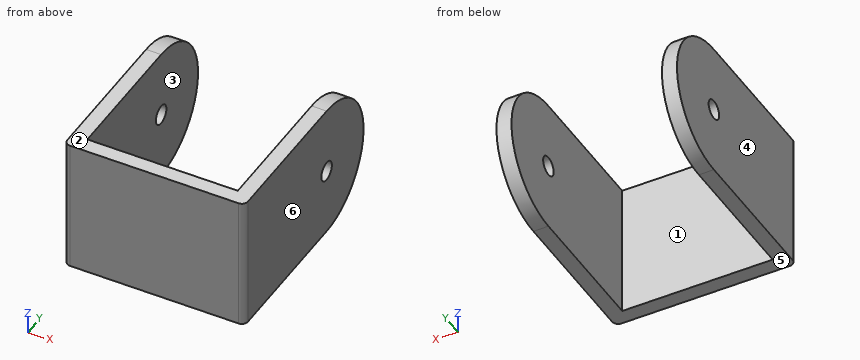
from build123d import *

# Parameters (mm, degrees)
BOSS_EXTRUDE1_DEPTH = 2.5
SKETCH2_W           = 27.5
SKETCH2_H           = 22.5
BOSS_EXTRUDE2_DEPTH = 2.5
SKETCH5_W           = 22.5
SKETCH5_H           = 25
BOSS_EXTRUDE3_DEPTH = 2.5
SKETCH6_R           = 1.6
CUT_EXTRUDE1_DEPTH  = 30
FILLET1_R           = 1


with BuildPart() as part:
    # Sketch1 → Boss-Extrude1 (new body)
    with BuildSketch(Plane(origin=(0, 0, 0), x_dir=(0, 0, -1), z_dir=(1, 0, 0))):
        with BuildLine():
            Line((-11.25, 0), (-11.25, -22.5))
            Line((-11.25, -22.5), (11.25, -22.5))
            Line((11.25, -22.5), (11.25, 0))
            ThreePointArc((11.25, 0), (0, 11.25), (-11.25, 0))
        make_face()
    extrude(amount=BOSS_EXTRUDE1_DEPTH)

    # Sketch2 → Boss-Extrude2 (add)
    with BuildSketch(Plane(origin=(0, -22.5, 0), x_dir=(-1, 0, 0), z_dir=(0, -1, 0))):
        with Locations((-13.75, 0)):
            Rectangle(SKETCH2_W, SKETCH2_H)
    extrude(amount=BOSS_EXTRUDE2_DEPTH)

    # Sketch5 → Boss-Extrude3 (add)
    with BuildSketch(Plane(origin=(27.5, 0, 0), x_dir=(0, 0, -1), z_dir=(1, 0, 0))):
        with BuildLine():
            ThreePointArc((-11.25, 0), (0, 11.25), (11.25, 0))
            Line((11.25, 0), (-11.25, 0))
        make_face()
        with Locations((0, -12.5)):
            Rectangle(SKETCH5_W, SKETCH5_H)
    extrude(amount=BOSS_EXTRUDE3_DEPTH)

    # Sketch6 → Cut-Extrude1 (cut)
    with BuildSketch(Plane(origin=(30, 0, 0), x_dir=(0, 0, -1), z_dir=(1, 0, 0))):
        Circle(SKETCH6_R)
    extrude(amount=-CUT_EXTRUDE1_DEPTH, mode=Mode.SUBTRACT)

    # Fillet1
    fillet1_edges = [part.edges().sort_by_distance(p)[0] for p in [
        (0, -25, 0),
        (30, -25, 0),
    ]]
    fillet(fillet1_edges, radius=FILLET1_R)


solid = part.part
Source: CAD feature listing. Evaluate the final solid. Frame: model axes, mm. Face numbers are marked on the shaded views. A direction names the side the tool comes from. Give positions to 0.01 mm unless a question says otherwise; leave off trailing zeros. Write each loop counter-clockwise with the first axis right and the second up, starting at its lowest first coordinate (ties: lowest second). Pieces come first, ordered by that corner, then holes. Notation, with made-up numbers: M -9.5,49.5 L 26.5,49.5 A16 cw 26.5,68.5 Z; hole C -34,-24.5 d1. An arc over 180 degrees is marked long. Return JSON: item names as keys, results as strings. Group by question number.
1) Pull-direction query (X, two-part tool) for the marked faces 3, 4, 5 and 6; classes: pulls with the +X half, pulls with the -X half, needs draft (parallel to the pull), parting line crosses it, or undercut.
2) Cut plane D-D, the plane y = 5.5. Output: boundary loops of the cut face in (x, z).
3) Cut plane C-C, the plane x = 11. Output: boundary loops of the cut face in (y, z).
4) Set-up query: the marked faces 1 and 2. Return all of +Z, -Z, +X, -X, +Y, -Y with unobstructed straight access to the full face (end or side cutting, diameter ignored); none if empty.
5) Cut plane A-A, the plane y = -7.5. Output: boundary loops of the cut face in (x, z).
6) Pin query (flat end, axial travel): P1, Ø3, axis at y = 0, z = 0, coming from the -X side. Return the tip coordinate at first contact, or that it passes through.
7) Material intervals for line 1 along X through (y, z) = (-11.5, -7.5); line 2 along Y through (x, z) = (28.8, 0); line 3 along Y through (x, z) = (7, 0.75), sorted ascending. Write a range as [from, to].
8) Cut plane B-B, the plane z = -9. Output: boundary loops of the cut face in (x, y), plus the area to 3 significant figures.
Recorded:
{
 "1": {"face 3": "undercut", "face 4": "pulls with the -X half", "face 5": "needs draft", "face 6": "pulls with the +X half"},
 "2": {"outline": "M 0,-9.81 L 2.5,-9.81 L 2.5,9.81 L 0,9.81 Z; M 27.5,-9.81 L 30,-9.81 L 30,9.81 L 27.5,9.81 Z"},
 "3": {"outline": "M -25,-11.25 L -22.5,-11.25 L -22.5,11.25 L -25,11.25 Z"},
 "4": {"face 1": "+Z, -Z, +Y", "face 2": "+Z, +X, -X, +Y, -Y"},
 "5": {"outline": "M 0,-11.25 L 2.5,-11.25 L 2.5,11.25 L 0,11.25 Z; M 27.5,-11.25 L 30,-11.25 L 30,11.25 L 27.5,11.25 Z"},
 "6": {"P1": "passes through"},
 "7": {"line 1": "x = [0, 2.5], [27.5, 30]", "line 2": "y = [-25, -1.6], [1.6, 11.25]", "line 3": "y = [-25, -22.5]"},
 "8": {"outline": "M 0,-24 A1 ccw 1,-25 L 29,-25 A1 ccw 30,-24 L 30,6.75 L 27.5,6.75 L 27.5,-22.5 L 2.5,-22.5 L 2.5,6.75 L 0,6.75 Z", "area": "221 mm²"}
}
